from build123d import *

# Parameters (mm, degrees)
F0_R     = 10.9982
F0_R_2   = 13.97
F1_DEPTH = 12.7


with BuildPart() as f1:
    # F0 (on Top) → F1 (new body)
    with BuildSketch(Plane.XY):
        with BuildLine():
            ThreePointArc((13.97, 32.4071533978), (12.4598818148, 38.7247672797), (8.2560064193, 43.6765481466))
            ThreePointArc((8.2560064193, 43.6765481466), (0, 44.45), (-8.2560064193, 43.6765481466))
            ThreePointArc((-8.2560064193, 43.6765481466), (-13.8783328045, 34.0048951062), (-10.600858317, 23.3086533597))
            ThreePointArc((-10.600858317, 23.3086533597), (1.6096047371, 18.5301914612), (12.4020690853, 25.9767893021))
            ThreePointArc((12.4020690853, 25.9767893021), (13.5723580324, 29.097773178), (13.97, 32.4071533978))
        make_face()
        with Locations((0, 32.4071533978)):
            Circle(F0_R, mode=Mode.SUBTRACT)
        with BuildLine():
            ThreePointArc((-8.2560064193, 43.6765481466), (0, 44.45), (8.2560064193, 43.6765481466))
            ThreePointArc((8.2560064193, 43.6765481466), (0, 46.3771533978), (-8.2560064193, 43.6765481466))
        make_face()
        with BuildLine():
            ThreePointArc((42.0354181068, -16.2035766989), (42.0147992276, -15.4448499046), (41.9530034542, -14.6883627804))
            ThreePointArc((41.9530034542, -14.6883627804), (38.4948291982, -22.225), (33.696997035, -28.9881853662))
            ThreePointArc((33.696997035, -28.9881853662), (39.7665731273, -23.8353439377), (42.0354181068, -16.2035766989))
        make_face()
        with BuildLine():
            ThreePointArc((33.696997035, -28.9881853662), (38.4948291982, -22.225), (41.9530034542, -14.6883627804))
            ThreePointArc((41.9530034542, -14.6883627804), (36.4931838712, -5.0620478891), (25.7444185967, -2.4277333028))
            ThreePointArc((25.7444185967, -2.4277333028), (15.6881084253, -9.7256831332), (15.4233394109, -22.1482168264))
            ThreePointArc((15.4233394109, -22.1482168264), (23.1681669233, -29.287071295), (33.696997035, -28.9881853662))
        make_face()
        with Locations((28.0654181068, -16.2035766989)):
            Circle(F0_R, mode=Mode.SUBTRACT)
        with BuildLine():
            ThreePointArc((15.4233394109, -22.1482168264), (15.6881084253, -9.7256831332), (25.7444185967, -2.4277333028))
            ThreePointArc((25.7444185967, -2.4277333028), (12.8005092874, 8.8280600033), (12.4020690853, 25.9767893021))
            ThreePointArc((12.4020690853, 25.9767893021), (1.6096047371, 18.5301914612), (-10.600858317, 23.3086533597))
            ThreePointArc((-10.600858317, 23.3086533597), (-11.9457670792, 8.1377589695), (-20.5888732511, -4.4026370321))
            ThreePointArc((-20.5888732511, -4.4026370321), (-15.8259689437, -9.4688321468), (-14.0954181068, -16.2035766989))
            ThreePointArc((-14.0954181068, -16.2035766989), (-14.4683809608, -19.410051531), (-15.5673552362, -22.4453172))
            ThreePointArc((-15.5673552362, -22.4453172), (-0.1187696418, -17.419026699), (15.4233394109, -22.1482168264))
        make_face()
        Circle(F0_R_2, mode=Mode.SUBTRACT)
        with BuildLine():
            ThreePointArc((-20.5888732511, -4.4026370321), (-34.1254839966, -3.6164204906), (-41.9530034542, -14.6883627804))
            ThreePointArc((-41.9530034542, -14.6883627804), (-38.4948291982, -22.225), (-33.696997035, -28.9881853662))
            ThreePointArc((-33.696997035, -28.9881853662), (-23.3231157764, -29.3440283124), (-15.5673552362, -22.4453172))
            ThreePointArc((-15.5673552362, -22.4453172), (-14.4683809608, -19.410051531), (-14.0954181068, -16.2035766989))
            ThreePointArc((-14.0954181068, -16.2035766989), (-15.8259689437, -9.4688321468), (-20.5888732511, -4.4026370321))
        make_face()
        with Locations((-28.0654181068, -16.2035766989)):
            Circle(F0_R, mode=Mode.SUBTRACT)
        with BuildLine():
            ThreePointArc((-33.696997035, -28.9881853662), (-38.4948291982, -22.225), (-41.9530034542, -14.6883627804))
            ThreePointArc((-41.9530034542, -14.6883627804), (-40.1637929977, -23.1885766989), (-33.696997035, -28.9881853662))
        make_face()
        Circle(F0_R_2)
        Circle(F0_R, mode=Mode.SUBTRACT)
    extrude(amount=F1_DEPTH)


solid = f1.part
The model under review builds one solid part; all positions refer to its coordinate system, in mm. Coordinates: 2 decimals unless noted, no trailing zeros. Write each loop counter-clockwise with the first axis right and the second up, starting at its lowest first coordinate (ties: lowest second). Pieces come first, ordered by that corner, then holes. Notation, with made-up numbers: (29, 71.25) -> (59, 71.25) arc R19 ccw to (59, 81.25) -> close; hole circle Ø11 at (56.5, -12.5). An arc over 180 degrees is marked (long way). Answer in a Markdown table with one row per item.
1. Clearance check with flat-ended pins moving along their axes: pin 1 Ø1 at (x, z) = (-33, 9.5) entering from -Y; pin 2 Ø12 at (x, y) = (-14, -18.5) entering from -Z; pin 3 Ø1.5 at (x, z) = (3, 9.5) entering from -Y; pin 4 Ø2 at (x, z) = (-10.5, 5.5) entering from +Y. State where each tip first meets the part, or that it passes through.
Answers below:
| item | result |
|---|---|
| pin 1 | stops at y = -29.45 |
| pin 2 | stops at z = 0 |
| pin 3 | stops at y = -17.66 |
| pin 4 | stops at y = 42.65 |
2. We need section A-A, the plane x = 5.5. State the section outline as (y, z) points.
Answers below:
| item | result |
|---|---|
| outline | (-17.95, 0) -> (-9.52, 0) -> (-9.52, 12.7) -> (-17.95, 12.7) -> close; (9.52, 0) -> (22.88, 0) -> (22.88, 12.7) -> (9.52, 12.7) -> close; (41.93, 0) -> (45.25, 0) -> (45.25, 12.7) -> (41.93, 12.7) -> close |
3. Draft analysis for pull direction X (two halves, no side actions). For faces 1 (the cylindrical face through (38.556, -12.9, 6.261)), 2 (the flat face through (3, -12, 0)), state which applies: +X half, -X half, draft (parallel to the pull), parting line (faces both ways), or undercut.
Answers below:
| item | result |
|---|---|
| face 1 | undercut |
| face 2 | draft |
4. We need section C-C, the plane z = 8.5. State the section outline as (x, y) points.
Answers below:
| item | result |
|---|---|
| outline | (-20.59, -4.4) arc R13.97 ccw (long way) to (-15.57, -22.45) arc R27.05 cw to (15.42, -22.15) arc R13.97 ccw (long way) to (25.74, -2.43) arc R21.23 cw to (12.4, 25.98) arc R13.97 ccw (long way) to (-10.6, 23.31) arc R29.9 cw to start; hole circle Ø22 at (-28.07, -16.2); hole circle Ø22 at (0, 0); hole circle Ø22 at (0, 32.41); hole circle Ø22 at (28.07, -16.2) |
5. We need section D-D, the plane x = 32. State the section outline as (y, z) points, and give its area (3 significant figures).
Answers below:
| item | result |
|---|---|
| outline | (-29.61, 0) -> (-26.47, 0) -> (-26.47, 12.7) -> (-29.61, 12.7) -> close; (-5.93, 0) -> (-2.8, 0) -> (-2.8, 12.7) -> (-5.93, 12.7) -> close |
| area | 79.6 mm^2 |
6. We need section B-B, the plane y = 0. State the section outline as (x, z) points, and give its area (3 significant figures).
Answers below:
| item | result |
|---|---|
| outline | (-16.41, 0) -> (-11, 0) -> (-11, 12.7) -> (-16.41, 12.7) -> close; (11, 0) -> (20.53, 0) -> (20.53, 12.7) -> (11, 12.7) -> close |
| area | 190 mm^2 |
7. Wall thickness on probe 1 along X at (y, z) = (-24.5, 4.75); probe 2 along Y at (x, z) = (-3.5, 5.5); probe 3 along Y at (x, z) = (8.5, 2.5): over which ranges is each line inside the solid? List them lowest first. Write a range as [from, to].
Answers below:
| item | result |
|---|---|
| probe 1 | x = [-39.31, -35.29], [-20.85, -16.83], [16.83, 20.85], [35.29, 39.31] |
| probe 2 | y = [-17.66, -10.43], [10.43, 21.98], [42.83, 45.93] |
| probe 3 | y = [-18.74, -6.98], [6.98, 25.43], [39.39, 43.49] |
